```python
from build123d import *

# Parameters (mm, degrees)
SKETCH1_R           = 53.5
BOSS_EXTRUDE1_DEPTH = 14.5
SKETCH2_R           = 49.5
CUT_EXTRUDE1_DEPTH  = 2.5
SKETCH3_R           = 10
CUT_EXTRUDE3_DEPTH  = 14.5
SKETCH6_R           = 53.5
SKETCH6_R_2         = 30
CUT_EXTRUDE8_DEPTH  = 10
SKETCH7_R           = 27.8
CUT_EXTRUDE9_DEPTH  = 5


with BuildPart() as part:
    # Sketch1 → Boss-Extrude1 (new body)
    with BuildSketch(Plane.XY):
        with Locations(Location((0, 0, 0), (0, 0, 180))):
            Circle(SKETCH1_R)
    extrude(amount=BOSS_EXTRUDE1_DEPTH)

    # Sketch2 → Cut-Extrude1 (cut)
    with BuildSketch(Plane.XY.offset(14.5)):
        Circle(SKETCH2_R)
    extrude(amount=-CUT_EXTRUDE1_DEPTH, mode=Mode.SUBTRACT)

    # Sketch3 → Cut-Extrude3 (cut)
    with BuildSketch(Plane.XY.offset(12)):
        Circle(SKETCH3_R)
    extrude(amount=-CUT_EXTRUDE3_DEPTH, mode=Mode.SUBTRACT)

    # Sketch6 → Cut-Extrude8 (cut)
    with BuildSketch(Plane(origin=(0, 0, 0), x_dir=(-1, 0, 0), z_dir=(0, 0, -1))):
        Circle(SKETCH6_R)
        Circle(SKETCH6_R_2, mode=Mode.SUBTRACT)
    extrude(amount=-CUT_EXTRUDE8_DEPTH, mode=Mode.SUBTRACT)

    # Sketch7 → Cut-Extrude9 (cut)
    with BuildSketch(Plane(origin=(0, 0, 0), x_dir=(-1, 0, 0), z_dir=(0, 0, -1))):
        Circle(SKETCH7_R)
    extrude(amount=-CUT_EXTRUDE9_DEPTH, mode=Mode.SUBTRACT)


solid = part.part
```
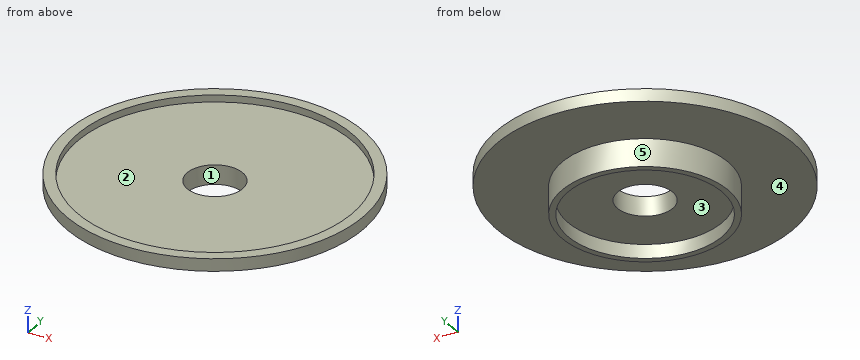
Check sheet for the modelled part. Datum: model origin and axes. Units: mm. Face numbers are marked on the shaded views. A direction names the side the tool comes from. Round coordinates to 2 decimals unless told otherwise and drop trailing zeros. Write each loop counter-clockwise with the first axis right and the second up, starting at its lowest first coordinate (ties: lowest second). Pieces come first, ordered by that corner, then holes. Notation, with made-up numbers: (72.25, 88) -> (125.25, 88) arc R23 cw to (125.25, 104) -> close; hole circle Ø8 at (62, 34.5). An arc over 180 degrees is marked (long way). One line per question, with ' | ' between items. Start each with the question number.
1. Release check for a two-part mould opening along X. For the marked faces 3, 4 and 5 record: +X half, -X half, draft (parallel to the pull), parting line (faces both ways), or undercut.
2. Sectioned sample at C-C, the plane x = 19.5. Record the cut outline in (y, z), then the cut area to 3 significant figures.
3. Set-up check for the marked faces 1 and 2: record each of +Z, -Z, +X, -X, +Y, -Y from which the full face is reachable in a straight line by a thin tool's end or side.
4. Depth check by flat-ended pin: pin 1 (3 mm diameter, centred on x = 38.5, y = 19.5, fed in from -Z); pin 2 (1 mm diameter, centred on x = -21.5, z = 13, fed in from -Y); pin 3 (5 mm diameter, centred on x = -33.5, y = 19.5, fed in from +Z). Enter the tip coordinate at first touch or a pass-through.
5. Scan lines: line 1 along X through (y, z) = (1, 1.5); line 2 along Y through (x, z) = (0, 3.85); line 3 along Y through (x, z) = (0, 13.6). Record each from-to range of solid material in increasing order. Write a range as from..to.
6. Sectioned sample at A-A, the plane x = 0. Record the cut outline in (y, z), then the cut area to 3 significant figures.
7. Sectioned sample at D-D, the plane z = 7.25. Record the cut outline in (x, y).
Taken from the geometry:
1) face 3: undercut | face 4: draft | face 5: parting line
2) outline: (-49.82, 10) -> (-22.8, 10) -> (-22.8, 0) -> (-19.81, 0) -> (-19.81, 5) -> (19.81, 5) -> (19.81, 0) -> (22.8, 0) -> (22.8, 10) -> (49.82, 10) -> (49.82, 14.5) -> (45.5, 14.5) -> (45.5, 12) -> (-45.5, 12) -> (-45.5, 14.5) -> (-49.82, 14.5) -> close | area: 479 mm^2
3) face 1: +Z, -Z | face 2: +Z
4) pin 1: stops at z = 10 | pin 2: stops at y = -49.21 | pin 3: stops at z = 12
5) line 1: x = -29.98..-27.78, 27.78..29.98 | line 2: y = -30..-27.8, 27.8..30 | line 3: y = -53.5..-49.5, 49.5..53.5
6) outline: (-53.5, 10) -> (-30, 10) -> (-30, 0) -> (-27.8, 0) -> (-27.8, 5) -> (-10, 5) -> (-10, 12) -> (-49.5, 12) -> (-49.5, 14.5) -> (-53.5, 14.5) -> close; (10, 5) -> (27.8, 5) -> (27.8, 0) -> (30, 0) -> (30, 10) -> (53.5, 10) -> (53.5, 14.5) -> (49.5, 14.5) -> (49.5, 12) -> (10, 12) -> close | area: 416 mm^2
7) outline: circle Ø60 at (0, 0); hole circle Ø20 at (0, 0)
